Autodesk Inventor part; units mm, degrees
ref_plane "YZ Plane" through (0, 0, 0) normal (1, 0, 0) x (0, 1, 0)
ref_plane "XZ Plane" through (0, 0, 0) normal (0, 1, 0) x (-1, 0, 0)
ref_plane "XY Plane" through (0, 0, 0) normal (0, 0, 1) x (1, 0, 0)
sketch "Sketch1" plane through (0, 0, 0) normal (0, 1, 0) x (-1, 0, 0)
  line L0 (-27, 0) -> (27, 0)
  line L1 (-27, 0) -> (-85.737, 70)
  line L2 (85.737, 70) -> (27, 0)
  line L3 (90.6672, 13.6467) -> (45.6523, -40)
  line L4 (45.6523, -40) -> (-45.6523, -40)
  line L5 (-45.6523, -40) -> (-90.6672, 13.6467)
  line L6 (0, 0) -> (0, -40) construction
  arc A0 (90.6672, 13.6467) -> (85.737, 70) centre (60.0255, 39.3582) ccw
  arc A1 (-85.737, 70) -> (-90.6672, 13.6467) centre (-60.0255, 39.3582) ccw
  point P0 (0, 70)
  dimension "d1" = 54
  dimension "d3" = 40
  dimension "d5" = 40
  dimension "d16" = 130
  dimension "d17" = 70
extrude "Extrusion1" add sketch "Sketch1" along normal blind 10
sketch "Sketch2" plane through (0, 0, 0) normal (0, -1, 0) x (1, 0, 0)
  line L0 (-27, 0) -> (27, 0)
  line L1 (-85.737, 70) -> (-27, 0)
  line L2 (-45.6523, -40) -> (-90.6672, 13.6467) construction
  line L3 (45.6523, -40) -> (-45.6523, -40) construction
  line L4 (90.6672, 13.6467) -> (45.6523, -40) construction
  line L5 (27, 0) -> (85.737, 70)
  line L6 (-97.6132, 53.039) -> (-36.3262, -20)
  line L7 (-36.3262, -20) -> (36.3262, -20)
  line L8 (36.3262, -20) -> (97.6132, 53.039)
  line L9 (-85.737, 70) -> (-27, 0)
  line L10 (27, 0) -> (85.737, 70)
  arc A0 (-85.737, 70) -> (-90.6672, 13.6467) centre (-60.0255, 39.3582) ccw
  arc A1 (90.6672, 13.6467) -> (85.737, 70) centre (60.0255, 39.3582) ccw
  point P0 (0, 0)
  dimension "d8" = 20
  dimension "d9" = 20
  dimension "d10" = 20
extrude "Extrusion2" cut sketch "Sketch2" against normal blind 3
fillet "Fillet1" radius 10 4 edges at (-85.737, 6.5, 70) (85.737, 6.5, 70) (-45.6523, 5, -40) (45.6523, 5, -40)
equation "\"d5\" = d3"
equation "\"d16\" = Лоток_угол"
equation "\"d9\" = d8"
equation "\"d10\" = d8"
properties part number "ДМС 045 держатель лотка"
Read the model definition and answer for the solid it produces. Units are mm, in the model's axes. A direction names the side the tool comes from. Coordinates: 2 decimals unless noted, no trailing zeros. Write each loop counter-clockwise with the first axis right and the second up, starting at its lowest first coordinate (ties: lowest second). Pieces come first, ordered by that corner, then holes. Notation, with made-up numbers: (-39.75, -10) -> (-14.75, -10) arc R21 cw to (-14.75, 13) -> close; hole circle Ø7 at (88, 14). An arc over 180 degrees is marked (long way). Write item = value, one per line.
(1) Section A-A on z = 2 is taken. Write down the section's boundary in (x, y), plus the area to 3 significant figures.
From the geometry:
outline = (-80.89, 0) -> (-54.79, 0) -> (-54.79, 3) -> (-28.68, 3) -> (-28.68, 10) -> (-80.89, 10) -> close; (28.68, 3) -> (54.79, 3) -> (54.79, 0) -> (80.89, 0) -> (80.89, 10) -> (28.68, 10) -> close
area = 888 mm2
(2) Section C-C on x = -12 is taken. Write down the section's boundary in (y, z).
From the geometry:
outline = (0, -40) -> (10, -40) -> (10, 0) -> (3, 0) -> (3, -20) -> (0, -20) -> close
(3) Given pin 1 Ø5 at (x, z) = (67, 31) entering from -Y; pin 2 Ø5.5 at (x, y) = (-1, 7) entering from +Z; pin 3 Ø1.5 at (y, z) = (8, 45.5) entering from +X, each flat-ended and moving along its own axis, determine where each tip first touches the part or whether it passes through.
From the geometry:
pin_1 = 3
pin_2 = 0
pin_3 = 99.66
(4) Section B-B on y = 5.5 is taken. Write down the section's boundary in (x, z).
From the geometry:
outline = (-94.48, 59.68) arc R40 ccw to (-90.67, 13.65) -> (-48.65, -36.43) arc R10 ccw to (-40.99, -40) -> (40.99, -40) arc R10 ccw to (48.65, -36.43) -> (90.67, 13.65) arc R40 ccw to (94.48, 59.68) arc R10 ccw to (78.21, 61.03) -> (27, 0) -> (-27, 0) -> (-78.21, 61.03) arc R10 ccw to start
(5) Which of the six approach directions +Z, -Z, +X, -X, +Y, -Y give full straight-line access (tool end or side, diameter ignored) to faces 5 (the face through (-52.96, 6.45, 30.94)), 6 (the face through (1, 10, -10)), 7 (the face through (66.54, 1.48, 16.01))?
From the geometry:
face_5 = +Z, +Y, -Y
face_6 = +Z, -Z, +X, -X, +Y
face_7 = +Z, -Y
(6) For a pull along X with two mould halves and no side action, classify faces 1 (the face through (0, 3, -3)), 2 (the face through (0, 0, -21)), 3 (the face through (86.559, 6.549, 64.573)), 4 (the face through (-45.16, 5.07, -39.09)) as +X half, -X half, draft (parallel to the pull), parting line (faces both ways), or undercut.
From the geometry:
face_1 = undercut
face_2 = draft
face_3 = undercut
face_4 = -X half
(7) Section D-D on z = 37 is taken. Write down the section's boundary in (x, y).
From the geometry:
outline = (-99.96, 0) -> (-84.15, 0) -> (-84.15, 3) -> (-58.05, 3) -> (-58.05, 10) -> (-99.96, 10) -> close; (58.05, 3) -> (84.15, 3) -> (84.15, 0) -> (99.96, 0) -> (99.96, 10) -> (58.05, 10) -> close
(8) Straight lines are drawn through the part: L1, parallel to Z at x = -25, y = 7; L2, parallel to Z at x = -2.5, y = 2.5; L3, parallel to Y at x = 17, z = -11. For each, find the intervals that lie inside material, in ascending order. Write a range as from..to.
From the geometry:
L1 = -40..0
L2 = -40..-20
L3 = 3..10
